Input: part model. Units: mm. Frame: model coordinates. Round coordinates to 2 decimals unless told otherwise and drop trailing zeros. Write each loop counter-clockwise with the first axis right and the second up, starting at its lowest first coordinate (ties: lowest second). Pieces come first, ordered by that corner, then holes. Notation, with made-up numbers: M -35,7.25 L 16,7.25 A15 cw 16,34.25 Z; hole C -17,-4.5 d5. An arc over 180 degrees is marked long. Write each question's results on one line, items separated by ' | '. Start each with the question number.
```python
from build123d import *

# Parameters (mm, degrees)
SKETCH_1_R          = 1.3
SKETCH_1_R_2        = 3.1
EXTRUDE_1_DEPTH     = 18
CUT_EXTRUDE_1_DEPTH = 39.778149269


with BuildPart() as part:
    # ｽｹｯﾁ1 → ﾎﾞｽ - 押し出し1 (new body)
    with BuildSketch(Plane.XY):
        with BuildLine():
            ThreePointArc((11.520520871, 18.842793666), (9.949769241, 24.020867845), (5.177628747, 21.470105609))
            ThreePointArc((5.177628747, 21.470105609), (0, 17.220935509), (-5.177628747, 21.470105609))
            ThreePointArc((-5.177628747, 21.470105609), (-9.949769241, 24.020867845), (-11.520520871, 18.842793666))
            ThreePointArc((-11.520520871, 18.842793666), (-12.177040277, 12.177040277), (-18.842793666, 11.520520871))
            ThreePointArc((-18.842793666, 11.520520871), (-24.020867845, 9.949769241), (-21.470105609, 5.177628747))
            ThreePointArc((-21.470105609, 5.177628747), (-17.220935509, 0), (-21.470105609, -5.177628747))
            ThreePointArc((-21.470105609, -5.177628747), (-24.020867845, -9.949769241), (-18.842793666, -11.520520871))
            ThreePointArc((-18.842793666, -11.520520871), (-12.177040277, -12.177040277), (-11.520520871, -18.842793666))
            ThreePointArc((-11.520520871, -18.842793666), (-9.949769241, -24.020867845), (-5.177628747, -21.470105609))
            ThreePointArc((-5.177628747, -21.470105609), (0, -17.220935509), (5.177628747, -21.470105609))
            ThreePointArc((5.177628747, -21.470105609), (9.949769241, -24.020867845), (11.520520871, -18.842793666))
            ThreePointArc((11.520520871, -18.842793666), (12.177040277, -12.177040277), (18.842793666, -11.520520871))
            ThreePointArc((18.842793666, -11.520520871), (24.020867845, -9.949769241), (21.470105609, -5.177628747))
            ThreePointArc((21.470105609, -5.177628747), (17.220935509, 0), (21.470105609, 5.177628747))
            ThreePointArc((21.470105609, 5.177628747), (24.020867845, 9.949769241), (18.842793666, 11.520520871))
            ThreePointArc((18.842793666, 11.520520871), (12.177040277, 12.177040277), (11.520520871, 18.842793666))
        make_face()
        with Locations((8.610377228, 20.787289482)):
            Circle(SKETCH_1_R, mode=Mode.SUBTRACT)
        with Locations((20.787289482, 8.610377228)):
            Circle(SKETCH_1_R, mode=Mode.SUBTRACT)
        with Locations((20.787289482, -8.610377228)):
            Circle(SKETCH_1_R, mode=Mode.SUBTRACT)
        with Locations((8.610377228, -20.787289482)):
            Circle(SKETCH_1_R, mode=Mode.SUBTRACT)
        with Locations((-8.610377228, -20.787289482)):
            Circle(SKETCH_1_R, mode=Mode.SUBTRACT)
        with Locations((-20.787289482, -8.610377228)):
            Circle(SKETCH_1_R, mode=Mode.SUBTRACT)
        with Locations((-20.787289482, 8.610377228)):
            Circle(SKETCH_1_R, mode=Mode.SUBTRACT)
        with Locations((-8.610377228, 20.787289482)):
            Circle(SKETCH_1_R, mode=Mode.SUBTRACT)
        with Locations((8.838834765, 8.838834765)):
            Circle(SKETCH_1_R, mode=Mode.SUBTRACT)
        with Locations((8.838834765, -8.838834765)):
            Circle(SKETCH_1_R, mode=Mode.SUBTRACT)
        with Locations((-8.838834765, -8.838834765)):
            Circle(SKETCH_1_R, mode=Mode.SUBTRACT)
        with Locations((-8.838834765, 8.838834765)):
            Circle(SKETCH_1_R, mode=Mode.SUBTRACT)
        with Locations((0, 6.5)):
            Circle(SKETCH_1_R, mode=Mode.SUBTRACT)
        with Locations((6.5, 0)):
            Circle(SKETCH_1_R, mode=Mode.SUBTRACT)
        with Locations((0, -6.5)):
            Circle(SKETCH_1_R, mode=Mode.SUBTRACT)
        with Locations((-6.5, 0)):
            Circle(SKETCH_1_R, mode=Mode.SUBTRACT)
        Circle(SKETCH_1_R_2, mode=Mode.SUBTRACT)
    extrude(amount=EXTRUDE_1_DEPTH)

    # ｽｹｯﾁ2 → ｶｯﾄ - 押し出し1 (cut, through all)
    with BuildSketch(Plane.XY.offset(18)):
        with BuildLine():
            ThreePointArc((3.249191362, 8.927079897), (0, 9.5), (-3.249191362, 8.927079897))
            ThreePointArc((-3.249191362, 8.927079897), (-7.126372473, 10.735039142), (-5.318413229, 14.612220253))
            ThreePointArc((-5.318413229, 14.612220253), (0, 15.55), (5.318413229, 14.612220253))
            ThreePointArc((5.318413229, 14.612220253), (7.126372473, 10.735039142), (3.249191362, 8.927079897))
        make_face()
        with BuildLine():
            ThreePointArc((8.927079897, 3.249191362), (10.735039142, 7.126372473), (14.612220253, 5.318413229))
            ThreePointArc((14.612220253, 5.318413229), (15.55, 0), (14.612220253, -5.318413229))
            ThreePointArc((14.612220253, -5.318413229), (10.735039142, -7.126372473), (8.927079897, -3.249191362))
            ThreePointArc((8.927079897, -3.249191362), (9.5, 0), (8.927079897, 3.249191362))
        make_face()
        with BuildLine():
            ThreePointArc((3.249191362, -8.927079897), (7.126372473, -10.735039142), (5.318413229, -14.612220253))
            ThreePointArc((5.318413229, -14.612220253), (0, -15.55), (-5.318413229, -14.612220253))
            ThreePointArc((-5.318413229, -14.612220253), (-7.126372473, -10.735039142), (-3.249191362, -8.927079897))
            ThreePointArc((-3.249191362, -8.927079897), (0, -9.5), (3.249191362, -8.927079897))
        make_face()
        with BuildLine():
            ThreePointArc((-8.927079897, -3.249191362), (-10.735039142, -7.126372473), (-14.612220253, -5.318413229))
            ThreePointArc((-14.612220253, -5.318413229), (-15.55, 0), (-14.612220253, 5.318413229))
            ThreePointArc((-14.612220253, 5.318413229), (-10.735039142, 7.126372473), (-8.927079897, 3.249191362))
            ThreePointArc((-8.927079897, 3.249191362), (-9.5, 0), (-8.927079897, -3.249191362))
        make_face()
    extrude(amount=-CUT_EXTRUDE_1_DEPTH, mode=Mode.SUBTRACT)


solid = part.part
```
1. Cut plane A-A on x = 0. Output: boundary loops of the cut face in (y, z).
2. Contact query for flat-ended pins moving along their axis: P1, Ø1.5, axis at x = -17, z = 11, coming from the +Y side; P2, Ø4, axis at x = 20.79, y = 8.61, coming from the -Z side; P3, Ø2, axis at y = 17.5, z = 15.5, coming from the +X side. Output: stop coordinate, or through.
3. Line query: L1, parallel to X at y = 21, z = 9; L2, parallel to X at y = -4, z = 8.75; L3, parallel to Y at x = -21.5, z = 8. Output: solid intervals per line, ascending. Write a range as from..to.
4. Draft query along X for faces 1 (the face through (-9.5, 0, 9.1)), 2 (the face through (-17.22, 0.1, 8.87)), 3 (the face through (-12.25, -12.106, 8.874)). Return one class per face: +X half, -X half, draft (parallel to the pull), parting line (faces both ways), or undercut.
5. Cut plane C-C on y = -6.5. Output: boundary loops of the cut face in (x, z).
Answers follow:
1) outline: M -17.22,0 L -15.55,0 L -15.55,18 L -17.22,18 Z; M -9.5,0 L -7.8,0 L -7.8,18 L -9.5,18 Z; M -5.2,0 L -3.1,0 L -3.1,18 L -5.2,18 Z; M 3.1,0 L 5.2,0 L 5.2,18 L 3.1,18 Z; M 7.8,0 L 9.5,0 L 9.5,18 L 7.8,18 Z; M 15.55,0 L 17.22,0 L 17.22,18 L 15.55,18 Z
2) P1: stops at y = 10.96 | P2: stops at z = 0 | P3: stops at x = 11.31
3) L1: x = -12.1..-9.89, -7.33..-5.06, 5.06..7.33, 9.89..12.1 | L2: x = -19.05..-15.03, -8.76..8.76, 15.03..19.05 | L3: y = -12.04..-9.7, -7.52..-5.18, 5.18..7.52, 9.7..12.04
4) face 1: undercut | face 2: -X half | face 3: undercut
5) outline: M -23.58,0 L -13.83,0 L -13.83,18 L -23.58,18 Z; M -9.71,0 L -1.3,0 L -1.3,18 L -9.71,18 Z; M 1.3,0 L 9.71,0 L 9.71,18 L 1.3,18 Z; M 13.83,0 L 23.58,0 L 23.58,18 L 13.83,18 Z
